```python
from build123d import *

# Parameters (mm, degrees)
SKETCH1_R           = 5
BASEHEAD_DEPTH      = 6
SKETCH2_R           = 3
BASEBODY_DEPTH      = 20
HEXAGONSOCKET_DEPTH = 3
TOPFILLET_R         = 0.75
CHAMFER1_SIZE       = 0.25
LPATTERN10_COUNT    = 31
LPATTERN10_PITCH    = 0.6498


with BuildPart() as part:
    # Sketch1 → BaseHead (new body)
    with BuildSketch(Plane(origin=(0, 0, 0), x_dir=(0, 0, -1), z_dir=(1, 0, 0))):
        Circle(SKETCH1_R)
    extrude(amount=BASEHEAD_DEPTH)

    # Sketch2 → BaseBody (add)
    with BuildSketch(Plane(origin=(6, 0, 0), x_dir=(0, 0, -1), z_dir=(1, 0, 0))):
        Circle(SKETCH2_R)
    extrude(amount=BASEBODY_DEPTH)

    # Sketch3 → HexagonSocket (cut)
    with BuildSketch(Plane(origin=(0, 0, 0), x_dir=(0, 0, -1), z_dir=(1, 0, 0))):
        Polygon((2.886751346, 0), (1.443375673, 2.5), (-1.443375673, 2.5), (-2.886751346, 0), (-1.443375673, -2.5), (1.443375673, -2.5), align=None)
    extrude(amount=HEXAGONSOCKET_DEPTH, mode=Mode.SUBTRACT)

    # Sketch4 → Cut-Revolve1 (revolve, cut)
    with BuildSketch(Plane(origin=(-4.19613823, 0.75, 0), x_dir=(-1, 0, 0), z_dir=(0, 0, 1))):
        Polygon((-7.19613823, 3.25), (-8.639513903, 0.75), (-7.19613823, 0.75), align=None)
    revolve(axis=Axis((0.838992387, 0, 0), (-1, 0, 0)), mode=Mode.SUBTRACT)

    # TopFillet
    topfillet_edges = [part.edges().sort_by_distance(p)[0] for p in [
        (0, 0, 5),
    ]]
    fillet(topfillet_edges, radius=TOPFILLET_R)

    # Chamfer1
    chamfer1_edges = [part.edges().sort_by_distance(p)[0] for p in [
        (26, 0, 3),
    ]]
    chamfer(chamfer1_edges, length=CHAMFER1_SIZE)

    # Sketch5 → Cut-Revolve10 (revolve, cut)
    with BuildSketch(Plane.XY):
        Polygon((25.75, 2.531047244), (26.02075, 3), (26.02075, 3.5415), (25.47925, 3.5415), (25.47925, 3), align=None)
    cut_revolve10 = revolve(axis=Axis((0, 0, 0), (1, 0, 0)), mode=Mode.SUBTRACT)

    # LPattern10: Cut-Revolve10 ×31
    with Locations(*[(-i * LPATTERN10_PITCH, 0, 0) for i in range(1, LPATTERN10_COUNT)]):
        add(cut_revolve10, mode=Mode.SUBTRACT)


solid = part.part
```
CAD build for the part. Positions are in the model's coordinates, mm. Coordinates: 2 decimals unless noted, no trailing zeros. Write each loop counter-clockwise with the first axis right and the second up, starting at its lowest first coordinate (ties: lowest second). Pieces come first, ordered by that corner, then holes.
(1) Flat gauge pins, fed straight in: pin 1 (0.6 mm diameter, centred on y = 2, z = 0.5, fed in from -X); pin 2 (1.5 mm diameter, centred on x = 6.5, z = -3, fed in from +Y); pin 3 (1.5 mm diameter, centred on x = 16.5, y = 3.5, fed in from -Z). Where does each tip first touch, or does it go through?
(2) Cut at A-A, the plane x = 1.75. List the corners of the cut face in (y, z), and give its area (3 significant figures).
(3) Drill centre lines: probe 1 along X at (y, z) = (-1.5, -3.25); probe 2 along Y at (x, z) = (6.05, 0). Where is each one in solid material? Low to high.
Geometry says:
1. pin 1: stops at x = 3.08
1. pin 2: stops at y = 4.36
1. pin 3: stops at z = -1.18
2. outline: circle Ø10 at (0, 0); hole (-2.5, -1.44) - (0, -2.89) - (2.5, -1.44) - (2.5, 1.44) - (0, 2.89) - (-2.5, 1.44) - close
2. area: 56.9 mm2
3. probe 1: x = 0 to 6
3. probe 2: y = -2.89 to 2.89
